```python
from build123d import *

# Parameters (mm, degrees)
SKETCH3_R           = 1.25
BOSS_EXTRUDE1_DEPTH = 1.35
FILLET1_R           = 5
FILLET2_R           = 2


with BuildPart() as part:
    # Sketch3 → Boss-Extrude1 (new body)
    with BuildSketch(Plane(origin=(0, 0, 0), x_dir=(1, 0, 0), z_dir=(0, 1, 0))):
        Polygon((-29.75, -55.35), (29.75, -55.35), (29.75, 30.244309853), (15.751559249, 44.95), (-15.731542027, 44.95), (-29.75, 30.263390376), align=None)
        with Locations(Location((13.515, 39.7, 0), (0, 0, 270))):
            Circle(SKETCH3_R, mode=Mode.SUBTRACT)
        with Locations(Location((-13.485, 39.7, 0), (0, 0, 270))):
            Circle(SKETCH3_R, mode=Mode.SUBTRACT)
        with Locations(Location((-24.5, 28.16, 0), (0, 0, 270))):
            Circle(SKETCH3_R, mode=Mode.SUBTRACT)
        with Locations(Location((-24.5, -29.84, 0), (0, 0, 270))):
            Circle(SKETCH3_R, mode=Mode.SUBTRACT)
        with Locations(Location((-24.085, -50.1, 0), (0, 0, 270))):
            Circle(SKETCH3_R, mode=Mode.SUBTRACT)
        with Locations(Location((24.5, -29.84, 0), (0, 0, 270))):
            Circle(SKETCH3_R, mode=Mode.SUBTRACT)
        with Locations(Location((24.015, -50.1, 0), (0, 0, 270))):
            Circle(SKETCH3_R, mode=Mode.SUBTRACT)
        with Locations(Location((24.5, 28.16, 0), (0, 0, 270))):
            Circle(SKETCH3_R, mode=Mode.SUBTRACT)
        Polygon((-19.25, -44.85), (19.25, -44.85), (19.25, 26.045705114), (11.249897805, 34.45), (-11.238457973, 34.45), (-19.25, 26.056609624), align=None, mode=Mode.SUBTRACT)
    extrude(amount=-BOSS_EXTRUDE1_DEPTH)

    # Fillet1
    fillet1_edges = [part.edges().sort_by_distance(p)[0] for p in [
        (29.75, -0.675, 55.35),
        (-29.75, -0.675, 55.35),
        (-29.75, -0.675, -30.263390376),
        (-15.731542027, -0.675, -44.95),
        (15.751559249, -0.675, -44.95),
        (29.75, -0.675, -30.244309853),
        (19.25, -0.675, -26.045705114),
        (-19.25, -0.675, -26.056609624),
        (-11.238457973, -0.675, -34.45),
        (11.249897805, -0.675, -34.45),
    ]]
    fillet(fillet1_edges, radius=FILLET1_R)

    # Fillet2
    fillet2_edges = [part.edges().sort_by_distance(p)[0] for p in [
        (19.25, -0.675, 44.85),
        (-19.25, -0.675, 44.85),
    ]]
    fillet(fillet2_edges, radius=FILLET2_R)


solid = part.part
```
Check sheet for the modelled part. Datum: model origin and axes. Units: mm. A direction names the side the tool comes from. Round coordinates to 2 decimals unless told otherwise and drop trailing zeros. Write each loop counter-clockwise with the first axis right and the second up, starting at its lowest first coordinate (ties: lowest second). Pieces come first, ordered by that corner, then holes. Notation, with made-up numbers: (18.5, 10) -> (49.5, 10) arc R28 ccw to (49.5, 49) -> close; hole circle Ø2 at (-7, 85.25). An arc over 180 degrees is marked (long way). One line per question, with ' | ' between items. Start each with the question number.
1. Sectioned sample at C-C, the plane y = -0.25. Count the separate pieces of the cut face and the enclosed holes in it, then the cut area to 3 significant figures.
2. Release check for a two-part mould opening along Z. For faces 3 (the face through (-20, 0, 4)), 4 (the face through (24.86, -0.67, 49.18)), 5 (the face through (-24.45, -0.67, -29.41)), 6 (the face through (22.88, -0.67, -37.46)) record: +Z half, -Z half, draft (parallel to the pull), parting line (faces both ways), or undercut.
3. Sectioned sample at D-D, the plane x = 11. Record the cut outline in (y, z).
4. Set-up check for faces 1 (the face through (28.25, -0.68, 53.92)), 2 (the face through (15.336, -0.666, -30.158)): record each of +Z, -Z, +X, -X, +Y, -Y from which the full face is reachable in a straight line by a thin tool's end or side.
5. Sectioned sample at A-A, the plane z = 29.84. Record the cut outline in (x, y), then the cut area to 3 significant figures.
6. Scan lines: line 1 along X through (y, z) = (-0.55, 50.1) (3 decimals); line 2 along X through (y, z) = (-0.5, -28.16); line 3 along X through (y, z) = (-1.1, 29.84). Record each from-to range of solid material in increasing order. Write a range as from..to.
7. Sectioned sample at B-B, the plane x = 4. Record the cut outline in (y, z).
Taken from the geometry:
1) separate pieces: 1 | enclosed holes: 9 | area: 2,730 mm^2
2) face 3: draft | face 4: undercut | face 5: undercut | face 6: -Z half
3) outline: (-1.35, -44.95) -> (0, -44.95) -> (0, -34.08) -> (-1.35, -34.08) -> close; (-1.35, 44.85) -> (0, 44.85) -> (0, 55.35) -> (-1.35, 55.35) -> close
4) face 1: +Z, +X, +Y, -Y | face 2: +Y, -Y
5) outline: (-29.75, -1.35) -> (-25.75, -1.35) -> (-25.75, 0) -> (-29.75, 0) -> close; (-23.25, -1.35) -> (-19.25, -1.35) -> (-19.25, 0) -> (-23.25, 0) -> close; (19.25, -1.35) -> (23.25, -1.35) -> (23.25, 0) -> (19.25, 0) -> close; (25.75, -1.35) -> (29.75, -1.35) -> (29.75, 0) -> (25.75, 0) -> close | area: 21.6 mm^2
6) line 1: x = -29.75..-25.335, -22.835..22.765, 25.265..29.75 | line 2: x = -29.75..-25.75, -23.25..-17.24, 17.24..23.25, 25.75..29.75 | line 3: x = -29.75..-25.75, -23.25..-19.25, 19.25..23.25, 25.75..29.75
7) outline: (-1.35, -44.95) -> (0, -44.95) -> (0, -34.45) -> (-1.35, -34.45) -> close; (-1.35, 44.85) -> (0, 44.85) -> (0, 55.35) -> (-1.35, 55.35) -> close
